from build123d import *

# Parameters (mm, degrees)
SKETCH_1_R          = 25
EXTRUDE_1_DEPTH     = 2
SKETCH_2_R          = 2.5
SKETCH_2_R_2        = 2
CUT_EXTRUDE_1_DEPTH = 2


with BuildPart() as part:
    # Эскиз1 → Бобышка-Вытянуть1 (new body)
    with BuildSketch(Plane(origin=(0, 0, 0), x_dir=(1, 0, 0), z_dir=(0, 1, 0))):
        with Locations(Location((0, 0, 0), (0, 0, 270))):
            Circle(SKETCH_1_R)
    extrude(amount=EXTRUDE_1_DEPTH)

    # Эскиз2 → Вырез-Вытянуть1 (cut)
    with BuildSketch(Plane(origin=(0, 2, 0), x_dir=(1, 0, 0), z_dir=(0, 1, 0))):
        with Locations(Location((0, 18, 0), (0, 0, 270))):
            Circle(SKETCH_2_R)
        with Locations(Location((15.588457268, 9, 0), (0, 0, 270))):
            Circle(SKETCH_2_R)
        with Locations(Location((15.588457268, -9, 0), (0, 0, 270))):
            Circle(SKETCH_2_R)
        with Locations(Location((0, -18, 0), (0, 0, 270))):
            Circle(SKETCH_2_R)
        with Locations(Location((-15.588457268, -9, 0), (0, 0, 270))):
            Circle(SKETCH_2_R)
        with Locations(Location((-15.588457268, 9, 0), (0, 0, 270))):
            Circle(SKETCH_2_R)
        with Locations(Location((-15.5, 0, 0), (0, 0, 270))):
            Circle(SKETCH_2_R_2)
        with Locations(Location((-7.75, 13.423393759, 0), (0, 0, 270))):
            Circle(SKETCH_2_R_2)
        with Locations(Location((7.75, 13.423393759, 0), (0, 0, 270))):
            Circle(SKETCH_2_R_2)
        with Locations(Location((15.5, 0, 0), (0, 0, 270))):
            Circle(SKETCH_2_R_2)
        with Locations(Location((7.75, -13.423393759, 0), (0, 0, 270))):
            Circle(SKETCH_2_R_2)
        with Locations(Location((-7.75, -13.423393759, 0), (0, 0, 270))):
            Circle(SKETCH_2_R_2)
    extrude(amount=-CUT_EXTRUDE_1_DEPTH, mode=Mode.SUBTRACT)


solid = part.part
Geometry check sheet. Reference: the model listing, model coordinates, mm. Coordinates: 2 decimals unless noted, no trailing zeros. Order: outer loops, then holes, each group sorted by start corner. A loop starts at its lowest first (then second) coordinate and runs counter-clockwise, first axis right, second up. Notation, with made-up numbers: (-30.75, 9) -> (-15.75, 9) arc R14 cw to (-15.75, 17) -> close; hole circle Ø11 at (-37, 56). An arc over 180 degrees is marked (long way). Use a Markdown table: item, result. Add a question column.
1. Cross-section at C-C (z = 18). Enter the section's corners in (x, y).
2. Cross-section at B-B (z = 0). Enter the section's corners in (x, y), and give its area (3 significant figures).
3. Material ranges on L1, parallel to Z at x = -17, y = 1; L2, parallel to X at y = 1.2, z = 0; L3, parallel to Z at x = -6, y = 1.65, recorded low to high.
4. Cross-section at A-A (x = 0). Enter the section's corners in (y, z).
5. Cross-section at D-D (y = 1.7). Give the number of separate pieces and of enclosed holes in the cut face, and give its area (3 significant figures).
6. Mould release check, pull along Z, two halves, no side actions. Record for faces 1 (the face through (0, 0, 0)), 2 (the face through (13.148, 1.014, -9.542)), 3 (the face through (7.509, 0.986, 23.846)): pulls with the +Z half, pulls with the -Z half, needs draft (parallel to the pull), parting line crosses it, or undercut.
7. Go/stop test with flat-tipped pins: pin 1 Ø2.5 at (x, z) = (7.75, 13.42) entering from -Y; pin 2 Ø1 at (x, y) = (-13, 0.5) entering from -Z; pin 3 Ø1 at (y, z) = (0.5, 20) entering from +X. Record where each tip stops, or that it passes through.
Filled sheet:
| question | item | result |
|---|---|---|
| 1 | outline | (-17.35, 0) -> (-2.5, 0) -> (-2.5, 2) -> (-17.35, 2) -> close; (2.5, 0) -> (17.35, 0) -> (17.35, 2) -> (2.5, 2) -> close |
| 2 | outline | (-25, 0) -> (-17.5, 0) -> (-17.5, 2) -> (-25, 2) -> close; (-13.5, 0) -> (13.5, 0) -> (13.5, 2) -> (-13.5, 2) -> close; (17.5, 0) -> (25, 0) -> (25, 2) -> (17.5, 2) -> close |
| 2 | area | 84.0 mm2 |
| 3 | L1 | -18.33 to -11.06, -6.94 to -1.32, 1.32 to 6.94, 11.06 to 18.33 |
| 3 | L2 | -25 to -17.5, -13.5 to 13.5, 17.5 to 25 |
| 3 | L3 | -24.27 to -14.39, -12.46 to 12.46, 14.39 to 24.27 |
| 4 | outline | (0, -25) -> (2, -25) -> (2, -20.5) -> (0, -20.5) -> close; (0, -15.5) -> (2, -15.5) -> (2, 15.5) -> (0, 15.5) -> close; (0, 20.5) -> (2, 20.5) -> (2, 25) -> (0, 25) -> close |
| 5 | separate pieces | 1 |
| 5 | enclosed holes | 12 |
| 5 | area | 1,770 mm2 |
| 6 | face 1 | needs draft |
| 6 | face 2 | undercut |
| 6 | face 3 | parting line crosses it |
| 7 | pin 1 | through |
| 7 | pin 2 | z = -21.65 |
| 7 | pin 3 | x = 15.64 |
